Design review of the part shown in the three views and the two pictorial views. Dimensions are in mm from the part's minimum x, y and z. Give positions to 0.01 mm unless a question says otherwise; leave off trailing zeros. Order: outer loops, then holes, each group sorted by start corner. A loop starts at its lowest first (then second) coordinate and runs counter-clockwise, first axis right, second up. Notation, with made-up numbers: (82, 85) - (99, 85) arc R23 cw to (99, 110) - close; hole circle Ø8 at (-38.5, 62.5). An arc over 180 degrees is marked (long way). Put each result on its own line as item: value.
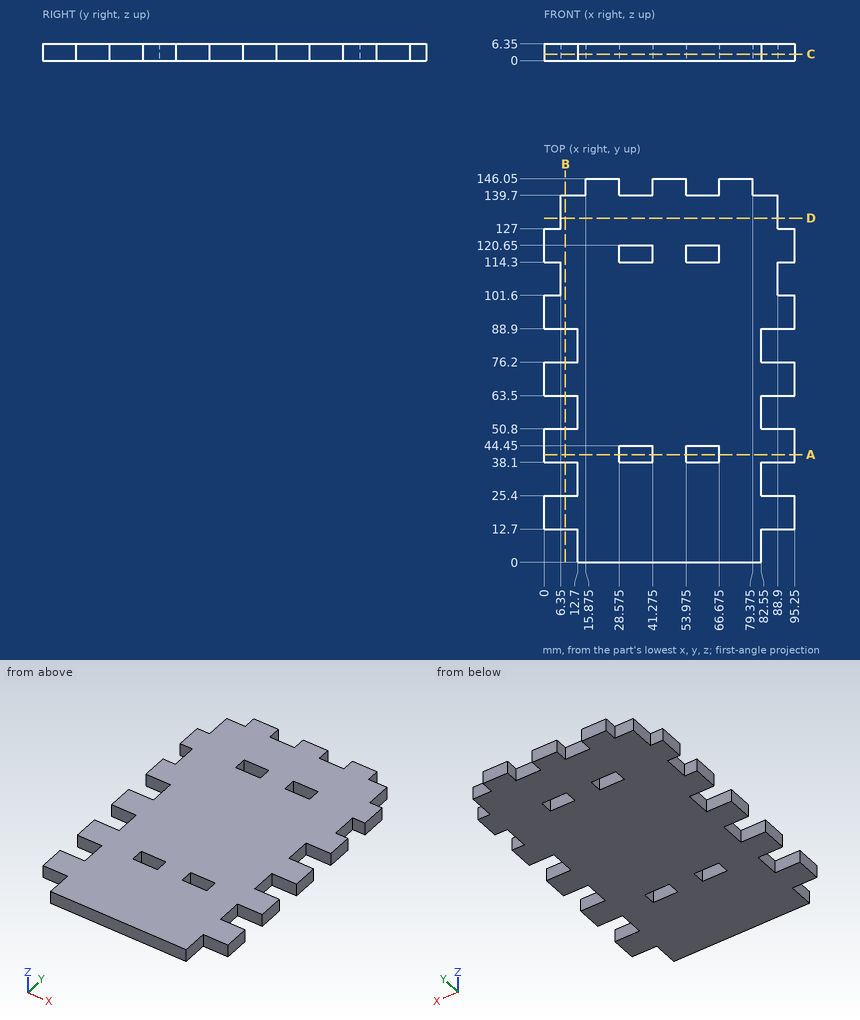
(1) Take a section at B-B, the plane x = 8. Write out the cut boundary in (y, z).
The answers:
outline: (12.7, 0) - (25.4, 0) - (25.4, 6.35) - (12.7, 6.35) - close; (38.1, 0) - (50.8, 0) - (50.8, 6.35) - (38.1, 6.35) - close; (63.5, 0) - (76.2, 0) - (76.2, 6.35) - (63.5, 6.35) - close; (88.9, 0) - (139.7, 0) - (139.7, 6.35) - (88.9, 6.35) - close
(2) Take a section at A-A, the plane y = 41. Write out the cut boundary in (x, z) (3 decimals), then the cut area to 3 significant figures.
The answers:
outline: (0, 0) - (28.575, 0) - (28.575, 6.35) - (0, 6.35) - close; (41.275, 0) - (53.975, 0) - (53.975, 6.35) - (41.275, 6.35) - close; (66.675, 0) - (95.25, 0) - (95.25, 6.35) - (66.675, 6.35) - close
area: 444 mm^2
(3) Take a section at D-D, the plane y = 131. Write out the cut boundary in (x, z), then the cut area to 3 significant figures.
The answers:
outline: (6.35, 0) - (88.9, 0) - (88.9, 6.35) - (6.35, 6.35) - close
area: 524 mm^2
(4) Wall thickness on L1, parallel to Y at x = 12.5, z = 3; L2, parallel to Y at x = 55, z = 4; L3, parallel to X at y = 44, z = 4.5 (3 decimals): over which ranges is each line inside the solid? List them lowest first.
The answers:
L1: 12.7 to 25.4, 38.1 to 50.8, 63.5 to 76.2, 88.9 to 139.7
L2: 0 to 38.1, 44.45 to 114.3, 120.65 to 139.7
L3: 0 to 28.575, 41.275 to 53.975, 66.675 to 95.25
(5) Clearance check with flat-ended pins moving along their axes: pin 1 Ø3 at (y, z) = (111, 4.5) entering from -X; pin 2 Ø1.9 at (y, z) = (80, 4) entering from -X; pin 3 Ø3 at (x, z) = (35, 2.5) entering from +Y. State where each tip first meets the part, or that it passes through.
The answers:
pin 1: x = 6.35
pin 2: x = 12.7
pin 3: y = 139.7
(6) Take a section at C-C, the plane z = 2.5. Count the separate pieces of the cut face and the enclosed holes in it, then the cut area to 3 significant figures.
The answers:
separate pieces: 1
enclosed holes: 4
area: 11,600 mm^2
